Geometry: final body of the model. Coordinates: model frame, mm. Face numbers are marked on the shaded views. A direction names the side the tool comes from. Give positions to 0.01 mm unless a question says otherwise; leave off trailing zeros. Write each loop counter-clockwise with the first axis right and the second up, starting at its lowest first coordinate (ties: lowest second). Pieces come first, ordered by that corner, then holes. Notation, with made-up numbers: M -38.75,39.5 L -1.75,39.5 A7 cw -1.75,52.5 Z; hole C -15,71.25 d10. An arc over 180 degrees is marked long. Use a Markdown table: item, result. Add a question column.
(1) Reachability of the marked faces 1 and 2 from +Z, -Z, +X, -X, +Y, -Y: full face, straight path, thin tool, end or side. Return the list, or none.
(2) Cut plane D-D (z = -6.75). Output: boundary loops of the cut face in (x, y) (3 decimals).
(3) Cut plane C-C (x = 2.85). Output: boundary loops of the cut face in (y, z) (3 decimals).
(4) Cut plane A-A (z = 0). Output: boundary loops of the cut face in (x, y) (3 decimals), plus the area to 3 significant figures.
(5) Material intervals for L1, parallel to Z at x = 1.9, y = 3 (3 decimals); L2, parallel to Z at x = 2.2, y = -0.5 (3 decimals); L3, parallel to Y at x = 1.1, z = 0.75 (3 decimals), sorted ascending.
(6) Pin query (flat end, axial travel): pin 1 Ø1.5 at (x, y) = (1, 1.5) entering from +Z. Return the tip coordinate at first contact, or that it passes through.
(7) Draft query along Y for the marked faces 3, 4 and 5. Return one class per face: released by +Y, released by -Y, zero draft, split by the parting line, or undercut.
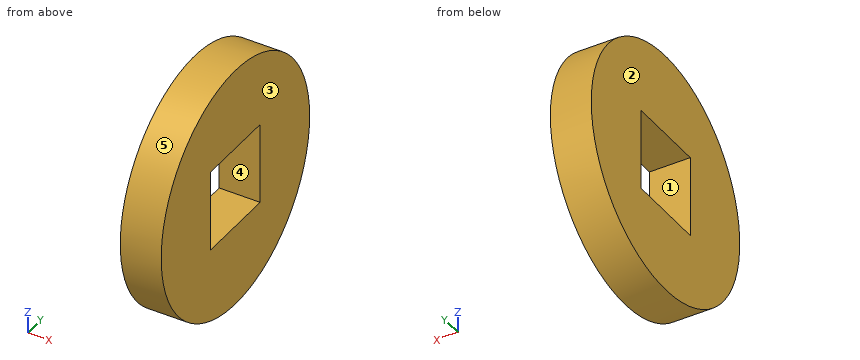
```python
from build123d import *

# Parameters (mm, degrees)
F0_R     = 9.525
F0_W     = 6.35
F0_H     = 6.35
F1_DEPTH = 3.175


with BuildPart() as f1:
    # F0 (on Right) → F1 (new body)
    with BuildSketch(Plane.YZ):
        Circle(F0_R)
        Rectangle(F0_W, F0_H, mode=Mode.SUBTRACT)
    extrude(amount=F1_DEPTH)


solid = f1.part
```
Answer list:
| question | item | result |
|---|---|---|
| 1 | face 1 | +X, -X |
| 1 | face 2 | +Z, -Z, -X, +Y, -Y |
| 2 | outline | M 0,-6.72 L 3.175,-6.72 L 3.175,6.72 L 0,6.72 Z |
| 3 | outline | C 0,0 d19.05; hole M -3.175,-3.175 L 3.175,-3.175 L 3.175,3.175 L -3.175,3.175 Z |
| 4 | outline | M 0,-9.525 L 3.175,-9.525 L 3.175,-3.175 L 0,-3.175 Z; M 0,3.175 L 3.175,3.175 L 3.175,9.525 L 0,9.525 Z |
| 4 | area | 40.3 mm² |
| 5 | L1 | -9.04 to -3.175, 3.175 to 9.04 |
| 5 | L2 | -9.512 to -3.175, 3.175 to 9.512 |
| 5 | L3 | -9.495 to -3.175, 3.175 to 9.495 |
| 6 | pin 1 | z = 9.5 |
| 7 | face 3 | zero draft |
| 7 | face 4 | undercut |
| 7 | face 5 | split by the parting line |
